```python
from build123d import *

# Parameters (mm, degrees)
SKETCH1_W           = 700
SKETCH1_H           = 120
BOSS_EXTRUDE1_DEPTH = 20
SKETCH2_W           = 700
SKETCH2_H           = 242
BOSS_EXTRUDE2_DEPTH = 20
BOSS_EXTRUDE3_DEPTH = 100
SKETCH4_R           = 50
CUT_EXTRUDE1_DEPTH  = 30
BOSS_EXTRUDE4_START = 50
SKETCH5_W           = 180
SKETCH5_H           = 165
SKETCH5_R           = 49.3285836
SKETCH5_R_2         = 50
BOSS_EXTRUDE4_DEPTH = 50
SKETCH7_R           = 60
CUT_EXTRUDE2_DEPTH  = 40
FILLET1_R           = 30
CHAMFER1_SIZE       = 30
SKETCH8_W           = 12
SKETCH8_H           = 50
BOSS_EXTRUDE5_DEPTH = 47.5
CIRPATTERN1_COUNT   = 6
SKETCH11_R          = 7.25
CUT_EXTRUDE3_DEPTH  = 40
SKETCH12_R          = 8.75
CUT_EXTRUDE4_DEPTH  = 40


with BuildPart() as part:
    # Sketch1 → Boss-Extrude1 (new body)
    with BuildSketch(Plane(origin=(0, 0, 0), x_dir=(1, 0, 0), z_dir=(0, 1, 0))):
        with Locations((0, -60)):
            Rectangle(SKETCH1_W, SKETCH1_H)
    extrude(amount=BOSS_EXTRUDE1_DEPTH)

    # Sketch2 → Boss-Extrude2 (add)
    with BuildSketch(Plane.XY):
        with Locations((0, 141)):
            Rectangle(SKETCH2_W, SKETCH2_H)
    extrude(amount=BOSS_EXTRUDE2_DEPTH)

    # Sketch3 → Boss-Extrude3 (add)
    with BuildSketch(Plane.XY.offset(20)):
        Polygon((350, 262), (-350, 262), (-350, 250), (-280, 250), (-280, 20), (-264, 20), (-264, 250), (264, 250), (264, 20), (280, 20), (280, 250), (350, 250), align=None)
    extrude(amount=BOSS_EXTRUDE3_DEPTH)

    # Sketch4 → Cut-Extrude1 (cut)
    with BuildSketch(Plane.XY.offset(20)):
        with Locations((-115, 150)):
            Circle(SKETCH4_R)
        with Locations((115, 150)):
            Circle(SKETCH4_R)
    extrude(amount=-CUT_EXTRUDE1_DEPTH, mode=Mode.SUBTRACT)

    # Sketch5 → Boss-Extrude4 (add)
    # profile 1 of 2: a face of its own
    with BuildSketch(Plane.XY.offset(20).offset(BOSS_EXTRUDE4_START)):
        with Locations((-115, 150)):
            Rectangle(SKETCH5_W, SKETCH5_H)
        with Locations((-115, 150)):
            Circle(SKETCH5_R, mode=Mode.SUBTRACT)
    # profile 2 of 2: a face of its own
    with BuildSketch(Plane.XY.offset(20).offset(BOSS_EXTRUDE4_START)):
        with Locations((115, 150)):
            Rectangle(SKETCH5_W, SKETCH5_H)
        with Locations((115, 150)):
            Circle(SKETCH5_R_2, mode=Mode.SUBTRACT)
    extrude(amount=-BOSS_EXTRUDE4_DEPTH)

    # Sketch7 → Cut-Extrude2 (cut)
    with BuildSketch(Plane.XY.offset(70)):
        with Locations((-115, 150)):
            Circle(SKETCH7_R)
        with Locations((115, 150)):
            Circle(SKETCH7_R)
    extrude(amount=-CUT_EXTRUDE2_DEPTH, mode=Mode.SUBTRACT)

    # Fillet1
    fillet1_edges = [part.edges().sort_by_distance(p)[0] for p in [
        (350, 256, 120),
        (-350, 256, 120),
        (350, 10, 120),
        (-350, 10, 120),
    ]]
    fillet(fillet1_edges, radius=FILLET1_R)

    # Chamfer1
    chamfer1_edges = [part.edges().sort_by_distance(p)[0] for p in [
        (-25, 67.5, 45),
        (-25, 232.5, 45),
        (-205, 232.5, 45),
        (-205, 67.5, 45),
        (205, 67.5, 45),
        (205, 232.5, 45),
        (25, 232.5, 45),
        (25, 67.5, 45),
    ]]
    chamfer(chamfer1_edges, length=CHAMFER1_SIZE)

    # Sketch8 → Boss-Extrude5 (add)
    with BuildSketch(Plane(origin=(0, 20, 0), x_dir=(1, 0, 0), z_dir=(0, 1, 0))):
        with Locations((-66, -45)):
            Rectangle(SKETCH8_W, SKETCH8_H)
        with Locations((66, -45)):
            Rectangle(SKETCH8_W, SKETCH8_H)
        with Locations((158, -45)):
            Rectangle(SKETCH8_W, SKETCH8_H)
        with Locations((-158, -45)):
            Rectangle(SKETCH8_W, SKETCH8_H)
    extrude(amount=BOSS_EXTRUDE5_DEPTH)

    # Sketch10 → M10 Tapped Hole1 (revolve, cut)
    with BuildSketch(Plane(origin=(-54.378221735, 185, 70), x_dir=(0, -1, 0), z_dir=(1, 0, 0))):
        Polygon((0, 0), (0, 30.053657631), (4.25, 27.5), (4.25, 0.650302214), (5.025, 0), align=None)
    m10_tapped_hole1 = revolve(axis=Axis((-54.378221735, 185, 76.35), (0, 0, -1)), mode=Mode.SUBTRACT)

    # CirPattern1: M10 Tapped Hole1 ×6 about axis
    cirpattern1_axis = Axis((-115, 150, 0), (0, 0, 1))
    for i in range(1, CIRPATTERN1_COUNT):
        add(m10_tapped_hole1.rotate(cirpattern1_axis, i * 360 / CIRPATTERN1_COUNT), mode=Mode.SUBTRACT)

    # Mirror1: M10 Tapped Hole1 across plane
    add(m10_tapped_hole1.mirror(Plane(origin=(0, 0, 0), x_dir=(0, 0, 1), z_dir=(1, 0, 0))), mode=Mode.SUBTRACT)

    # Mirror1 copy 1 sketch → Mirror1 copy 1 (revolve, cut)
    with BuildSketch(Plane(origin=(115, 220, 70), x_dir=(-0.8660254037844386, -0.5000000000000001, 0), z_dir=(-0.5000000000000001, 0.8660254037844386, 0))):
        Polygon((0, 0), (0, -30.053657631), (4.25, -27.5), (4.25, -0.650302214), (5.025, 0), align=None)
    revolve(axis=Axis((115, 220, 76.35), (0, 0, 1)), mode=Mode.SUBTRACT)

    # Mirror1 copy 2 sketch → Mirror1 copy 2 (revolve, cut)
    with BuildSketch(Plane(origin=(175.621778265, 185, 70), x_dir=(-0.8660254037844387, 0.4999999999999998, 0), z_dir=(0.4999999999999998, 0.8660254037844387, 0))):
        Polygon((0, 0), (0, -30.053657631), (4.25, -27.5), (4.25, -0.650302214), (5.025, 0), align=None)
    revolve(axis=Axis((175.621778265, 185, 76.35), (0, 0, 1)), mode=Mode.SUBTRACT)

    # Mirror1 copy 3 sketch → Mirror1 copy 3 (revolve, cut)
    with BuildSketch(Plane(origin=(175.621778265, 115, 70), x_dir=(0, 1, 0), z_dir=(1, 0, 0))):
        Polygon((0, 0), (0, -30.053657631), (4.25, -27.5), (4.25, -0.650302214), (5.025, 0), align=None)
    revolve(axis=Axis((175.621778265, 115, 76.35), (0, 0, 1)), mode=Mode.SUBTRACT)

    # Mirror1 copy 4 sketch → Mirror1 copy 4 (revolve, cut)
    with BuildSketch(Plane(origin=(115, 80, 70), x_dir=(0.8660254037844384, 0.5000000000000004, 0), z_dir=(0.5000000000000004, -0.8660254037844384, 0))):
        Polygon((0, 0), (0, -30.053657631), (4.25, -27.5), (4.25, -0.650302214), (5.025, 0), align=None)
    revolve(axis=Axis((115, 80, 76.35), (0, 0, 1)), mode=Mode.SUBTRACT)

    # Mirror1 copy 5 sketch → Mirror1 copy 5 (revolve, cut)
    with BuildSketch(Plane(origin=(54.378221735, 115, 70), x_dir=(0.8660254037844386, -0.5000000000000001, 0), z_dir=(-0.5000000000000001, -0.8660254037844386, 0))):
        Polygon((0, 0), (0, -30.053657631), (4.25, -27.5), (4.25, -0.650302214), (5.025, 0), align=None)
    revolve(axis=Axis((54.378221735, 115, 76.35), (0, 0, 1)), mode=Mode.SUBTRACT)

    # Sketch11 → Cut-Extrude3 (cut)
    with BuildSketch(Plane.XY.offset(20)):
        with Locations((330, 212)):
            Circle(SKETCH11_R)
        with Locations((330, 162)):
            Circle(SKETCH11_R)
        with Locations((330, 100)):
            Circle(SKETCH11_R)
        with Locations((330, 50)):
            Circle(SKETCH11_R)
    cut_extrude3 = extrude(amount=-CUT_EXTRUDE3_DEPTH, mode=Mode.SUBTRACT)

    # Sketch12 → Cut-Extrude4 (cut)
    with BuildSketch(Plane(origin=(0, 20, 0), x_dir=(1, 0, 0), z_dir=(0, 1, 0))):
        with Locations(Location((311.966460743, -50, 0), (0, 0, 270))):
            Circle(SKETCH12_R)
        with Locations(Location((311.966460743, -100, 0), (0, 0, 270))):
            Circle(SKETCH12_R)
        with Locations(Location((192.081589636, -40.105889272, 0), (0, 0, 270))):
            Circle(SKETCH12_R)
        with Locations(Location((191.966460743, -106.780261963, 0), (0, 0, 270))):
            Circle(SKETCH12_R)
        with Locations(Location((12.081589636, -40.105889272, 0), (0, 0, 270))):
            Circle(SKETCH12_R)
        with Locations(Location((12.081589636, -100.343403493, 0), (0, 0, 270))):
            Circle(SKETCH12_R)
    cut_extrude4 = extrude(amount=-CUT_EXTRUDE4_DEPTH, mode=Mode.SUBTRACT)

    # Mirror3: Cut-Extrude3, Cut-Extrude4 across plane
    add(cut_extrude3.mirror(Plane(origin=(0, 0, 0), x_dir=(0, 0, 1), z_dir=(1, 0, 0))), mode=Mode.SUBTRACT)
    add(cut_extrude4.mirror(Plane(origin=(0, 0, 0), x_dir=(0, 0, 1), z_dir=(1, 0, 0))), mode=Mode.SUBTRACT)


solid = part.part
```
Can you work these out from the model? Positions are in its coordinate system, mm. A direction names the side the tool comes from. Coordinates: 2 decimals unless noted, no trailing zeros. Write each loop counter-clockwise with the first axis right and the second up, starting at its lowest first coordinate (ties: lowest second). Pieces come first, ordered by that corner, then holes. Notation, with made-up numbers: M -8.75,-37 L 1.25,-37 A18 cw 1.25,-4 Z; hole C 84.5,-29.5 d5. An arc over 180 degrees is marked long. Write item = value, one per line. Start each with the question number.
Q1. If I drill on L1, parallel to Y at x = -330, z = 15.5; L2, parallel to X at y = 9, z = 50; L3, parallel to X at y = 23.5, z = 53.5, over which ranges is the centre line in solid material (lowest first)? Write a range as [from, to].
Q2. I'm going to push flat-ended pins straight in: pin 1 (8.5 mm diameter, centred on x = -330, y = 162, fed in from +Z); pin 2 (2 mm diameter, centred on y = 115.5, z = 22, fed in from +X); pin 3 (1.5 mm diameter, centred on y = 45.5, z = 68, fed in from -X); pin 4 (7 mm diameter, centred on x = -175.62, y = 115, fed in from +Z). Where does each tip first touch, or does it pass through?
Q3. Thinking about a two-plate mould opening in X: for faces 1 (the face through (350, 121, 15)), 2 (the face through (5, 262, 59)), 3 (the face through (-14.71, 10.14, 108.69)), which applies, released by +X, released by -X, zero draft, split by the parting line, or undercut?
Q4. If we section it at B-B, the plane x = -330: Write out the boundary of the cut face in (y, z), then the cut area to 3 significant figures.
Q5. If we section it at A-A, the plane z = 78: Write out the boundary of the cut face in (x, y).
Q6. If we section it at C-C, the plane y = 50: State how many separate pieces and enclosed holes the cut face has, then the cut area to 3 significant figures.
Q7. On a 3-axis mill with a long thin cutter (end or side, diameter ignored), from which of +Z, -Z, +X, -X, +Y, -Y can I reach the whole of each face in a straight line? I mean faces 4 (the face through (315, 20, 69)), 5 (the face through (-315, 137, 20)), 6 (the face through (60, 43, 45)). Say none if no direction works.
Check sheet entries:
q1.L1 = [0, 42.75], [57.25, 92.75], [107.25, 154.75], [169.25, 204.75], [219.25, 262]
q1.L2 = [-350, -320.72], [-303.22, 303.22], [320.72, 350]
q1.L3 = [-280, -264], [-164, -152], [-72, -60], [60, 72], [152, 164], [264, 280]
q2.pin_1 = through
q2.pin_2 = 280
q2.pin_3 = -280
q2.pin_4 = 42.05
q3.face_1 = released by +X
q3.face_2 = zero draft
q3.face_3 = undercut
q4.outline = M 0,0 L 42.75,0 L 42.75,20 L 20,20 L 20,118.28 L 0,118.28 Z; M 57.25,0 L 92.75,0 L 92.75,20 L 57.25,20 Z; M 107.25,0 L 154.75,0 L 154.75,20 L 107.25,20 Z; M 169.25,0 L 204.75,0 L 204.75,20 L 169.25,20 Z; M 219.25,0 L 262,0 L 262,118.28 L 250,118.28 L 250,20 L 219.25,20 Z
q4.area = 7,230 mm²
q5.outline = M -350,0 L 350,0 L 350,20 L 280,20 L 280,250 L 350,250 L 350,262 L -350,262 L -350,250 L -280,250 L -280,20 L -350,20 Z; hole M -264,20 L 264,20 L 264,250 L -264,250 Z
q6.separate_pieces = 3
q6.enclosed_holes = 0
q6.area = 19,000 mm²
q7.face_4 = +Z, +X
q7.face_5 = +Z, -X
q7.face_6 = +Z
